Input: part model. Units: mm. Frame: model coordinates. A direction names the side the tool comes from. Give positions to 0.01 mm unless a question says otherwise; leave off trailing zeros. Order: outer loops, then holes, each group sorted by start corner. A loop starts at its lowest first (then second) coordinate and runs counter-clockwise, first axis right, second up. Notation, with made-up numbers: (10.5, 18) - (22.5, 18) arc R14 ccw to (22.5, 30) - close; hole circle Ø6 at (13, 20.25). An arc over 180 degrees is marked (long way). Answer in a Markdown table with one row per item. Add a question column.
from build123d import *

# Parameters (mm, degrees)
SKETCH1_W           = 40
SKETCH1_H           = 40
BOSS_EXTRUDE2_DEPTH = 10
SKETCH7_R           = 12.5
BOSS_EXTRUDE3_DEPTH = 11
CHAMFER4_SIZE       = 4
SKETCH10_R          = 4
CUT_EXTRUDE2_DEPTH  = 1
SKETCH11_R          = 2.5
CUT_EXTRUDE3_DEPTH  = 2
FILLET2_R           = 10
FILLET3_R           = 10
FILLET4_R           = 10
FILLET5_R           = 10
CUT_EXTRUDE4_DEPTH  = 1.3
BOSS_EXTRUDE5_DEPTH = 1
SKETCH16_R          = 1.490769086
BOSS_EXTRUDE6_DEPTH = 1
SKETCH17_R          = 1.318486688
CUT_EXTRUDE5_DEPTH  = 1


with BuildPart() as part:
    # Sketch1 → Boss-Extrude2 (new body)
    with BuildSketch(Plane.XY):
        with Locations((12.211538462, -8.365384615)):
            Rectangle(SKETCH1_W, SKETCH1_H)
    extrude(amount=-BOSS_EXTRUDE2_DEPTH)

    # Sketch7 → Boss-Extrude3 (add)
    with BuildSketch(Plane(origin=(0, 0, -10), x_dir=(-1, 0, 0), z_dir=(0, 0, -1))):
        with Locations((-12.211538462, -8.365384615)):
            Circle(SKETCH7_R)
    extrude(amount=BOSS_EXTRUDE3_DEPTH)

    # Chamfer4
    chamfer4_edges = [part.edges().sort_by_distance(p)[0] for p in [
        (24.711538462, -8.365384615, -21),
    ]]
    chamfer(chamfer4_edges, length=CHAMFER4_SIZE)

    # Sketch10 → Cut-Extrude2 (cut)
    with BuildSketch(Plane(origin=(0, 0, -21), x_dir=(-1, 0, 0), z_dir=(0, 0, -1))):
        with Locations((-12.126772213, -8.563172529)):
            Circle(SKETCH10_R)
    extrude(amount=-CUT_EXTRUDE2_DEPTH, mode=Mode.SUBTRACT)

    # Sketch11 → Cut-Extrude3 (cut)
    with BuildSketch(Plane.XY):
        with Locations((-3.809282546, 7.542414728)):
            Circle(SKETCH11_R)
    extrude(amount=-CUT_EXTRUDE3_DEPTH, mode=Mode.SUBTRACT)

    # Fillet2
    fillet2_edges = [part.edges().sort_by_distance(p)[0] for p in [
        (32.211538462, 11.634615385, -5),
    ]]
    fillet(fillet2_edges, radius=FILLET2_R)

    # Fillet3
    fillet3_edges = [part.edges().sort_by_distance(p)[0] for p in [
        (-7.788461538, 11.634615385, -5),
    ]]
    fillet(fillet3_edges, radius=FILLET3_R)

    # Fillet4
    fillet4_edges = [part.edges().sort_by_distance(p)[0] for p in [
        (-7.788461538, -28.365384615, -5),
    ]]
    fillet(fillet4_edges, radius=FILLET4_R)

    # Fillet5
    fillet5_edges = [part.edges().sort_by_distance(p)[0] for p in [
        (32.211538462, -28.365384615, -5),
    ]]
    fillet(fillet5_edges, radius=FILLET5_R)

    # Sketch13 → Cut-Extrude4 (cut)
    with BuildSketch(Plane(origin=(0, 11.634615385, 0), x_dir=(1, 0, 0), z_dir=(0, 1, 0))):
        with BuildLine():
            Line((3.30309253, 4.642088904), (8.298895956, 4.642088904))
            ThreePointArc((8.298895956, 4.642088904), (8.582742042, 5.327353975), (8.298895956, 6.012619047))
            Line((8.298895956, 6.012619047), (3.30309253, 6.012619047))
            ThreePointArc((3.30309253, 6.012619047), (3.019246443, 5.327353975), (3.30309253, 4.642088904))
        make_face()
    extrude(amount=-CUT_EXTRUDE4_DEPTH, mode=Mode.SUBTRACT)

    # Sketch14 → Boss-Extrude5 (add)
    with BuildSketch(Plane(origin=(0, 10.334615385, 0), x_dir=(1, 0, 0), z_dir=(0, 1, 0))):
        with BuildLine():
            Line((4.275726825, 5.482091249), (7.237840361, 5.482091249))
            ThreePointArc((7.237840361, 5.482091249), (7.33855994, 5.238932676), (7.237840361, 4.995774102))
            Line((7.237840361, 4.995774102), (4.275726825, 4.995774102))
            ThreePointArc((4.275726825, 4.995774102), (4.175007246, 5.238932676), (4.275726825, 5.482091249))
        make_face()
    extrude(amount=BOSS_EXTRUDE5_DEPTH)

    # Sketch16 → Boss-Extrude6 (add)
    with BuildSketch(Plane(origin=(0, 11.634615385, 0), x_dir=(1, 0, 0), z_dir=(0, 1, 0))):
        with Locations(Location((17.198709177, 5.253755482, 0), (0, 0, 270))):
            Circle(SKETCH16_R)
    extrude(amount=BOSS_EXTRUDE6_DEPTH)

    # Sketch17 → Cut-Extrude5 (cut)
    with BuildSketch(Plane(origin=(0, 0, -20), x_dir=(-1, 0, 0), z_dir=(0, 0, -1))):
        with Locations((-12.126772213, -8.563172529)):
            Circle(SKETCH17_R)
    extrude(amount=-CUT_EXTRUDE5_DEPTH, mode=Mode.SUBTRACT)


solid = part.part
Q1. Section A-A, the plane z = -8.5. Return loops of the section in (x, y).
Q2. Section D-D, the plane z = -17.5. Return loops of the section in (x, y).
Q3. Line query: probe 1 along Z at (x, y) = (6, -26); probe 2 along Y at (x, z) = (12.5, -13.5); probe 3 along Y at (x, z) = (13.5, -3). Output: solid intervals per line, ascending.
Q4. Pull-direction query (Y, two-part tool) for faces 1 (the cylindrical face through (15.075, -5.86, -20.507)), 2 (the cylindrical face through (-4.937, -25.358, -5.07)), 3 (the cylindrical face through (15.743, 12.128, -5.577)); classes: +Y half, -Y half, draft (parallel to the pull), parting line (faces both ways), or undercut.
Q5. Section C-C, the plane y = 8.5. Return loops of the section in (x, z).
Q6. Access query for faces 4 (the flat face through (6, 11, -4.642)), 5 (the flat face through (10, -9, -20)), 6 (the flat face through (12, -4, -21)). Directions: +Z, -Z, +X, -X, +Y, -Y. A direction counts if a zero-diameter tool reaches every point of the face in a straight line with its end or side. Return the directions, or none.
Q7. Section B-B, the plane x = -2.5. Return loops of the section in (y, z), then the cut area to 3 significant figures.
Q8. Contact query for flat-ended pins moving along their axis: P1, Ø3.5, axis at x = 12.13, y = -8.56, coming from the -Z side; P2, Ø0.7, axis at x = 6.5, y = 11, coming from the -Z side; P3, Ø4, axis at x = 9.5, z = -14.5, coming from the +Y side; P4, Ø5, axis at y = 8, z = -17, coming from the -X side. Output: stop coordinate, or through.
Computed:
| question | item | result |
|---|---|---|
| 1 | outline | (-7.79, -18.37) arc R10 ccw to (2.21, -28.37) - (22.21, -28.37) arc R10 ccw to (32.21, -18.37) - (32.21, 1.63) arc R10 ccw to (22.21, 11.63) - (2.21, 11.63) arc R10 ccw to (-7.79, 1.63) - close |
| 2 | outline | circle Ø24 at (12.21, -8.37) |
| 3 | probe 1 | z = -10 to 0 |
| 3 | probe 2 | y = -20.86 to 4.13 |
| 3 | probe 3 | y = -28.37 to 11.63 |
| 4 | face 1 | undercut |
| 4 | face 2 | -Y half |
| 4 | face 3 | draft |
| 5 | outline | (-5.06, -10) - (29.48, -10) - (29.48, 0) - (-5.06, 0) - close |
| 6 | face 4 | +Y |
| 6 | face 5 | -Z |
| 6 | face 6 | -Z, +X, -X, +Y, -Y |
| 7 | outline | (-27.19, -10) - (10.46, -10) - (10.46, 0) - (-27.19, 0) - close |
| 7 | area | 376 mm^2 |
| 8 | P1 | stops at z = -20 |
| 8 | P2 | stops at z = -10 |
| 8 | P3 | stops at y = 4.11 |
| 8 | P4 | passes through |
